from build123d import *

# Parameters (mm, degrees)
FILLET1_R     = 1
CHAMFER1_SIZE = 1


with BuildPart() as part:
    # Sketch1 → Revolve1 (revolve)
    with BuildSketch(Plane(origin=(0, 0, 0), x_dir=(0, 0, -1), z_dir=(1, 0, 0)), mode=Mode.PRIVATE) as revolve1_sk:
        with BuildLine():
            Line((-55, 0), (358, 0))
            Line((358, 0), (358, 30.75))
            ThreePointArc((358, 30.75), (357.69848481, 34.992640687), (356.8, 39.15))
            Line((356.8, 39.15), (331.5, 40.033495468))
            Line((331.5, 40.033495468), (331.5, 42.5))
            Line((331.5, 42.5), (318.5, 42.5))
            Line((318.5, 42.5), (318.5, 65))
            Line((318.5, 65), (200.002907484, 65))
            Line((200.002907484, 65), (200.002907484, 55))
            Line((200.002907484, 55), (148, 55))
            Line((148, 55), (148, 66))
            Line((148, 66), (80, 66))
            Line((80, 66), (80, 63))
            Line((80, 63), (74, 63))
            Line((74, 63), (74, 66))
            Line((74, 66), (57, 66))
            Line((57, 66), (57, 65))
            Line((57, 65), (42, 65))
            Line((42, 65), (42, 47))
            Line((42, 47), (22, 45.5))
            Line((22, 45.5), (2, 45.5))
            Line((2, 45.5), (2, 22.5))
            Line((2, 22.5), (0, 22.5))
            Line((0, 22.5), (0, 17.5))
            Line((0, 17.5), (-55, 17.5))
            Line((-55, 17.5), (-55, 0))
        make_face()
    revolve(revolve1_sk.sketch.rotate(Axis((0, 0, 61.708002771), (0, 0, -1)), 90), axis=Axis((0, 0, 61.708002771), (0, 0, -1)))

    # Fillet1
    fillet1_edges = [part.edges().sort_by_distance(p)[0] for p in [
        (-39.15, 0, -356.8),
    ]]
    fillet(fillet1_edges, radius=FILLET1_R)

    # Chamfer1
    chamfer1_edges = [part.edges().sort_by_distance(p)[0] for p in [
        (-17.5, 0, 55),
    ]]
    chamfer(chamfer1_edges, length=CHAMFER1_SIZE)


solid = part.part
Geometry check sheet. Reference: the model listing, model coordinates, mm. A direction names the side the tool comes from. Round coordinates to 2 decimals unless told otherwise and drop trailing zeros. Order: outer loops, then holes, each group sorted by start corner. A loop starts at its lowest first (then second) coordinate and runs counter-clockwise, first axis right, second up. Notation, with made-up numbers: M -10.5,13 L 48.5,13 A31 ccw 48.5,43 Z; hole C -2,19.5 d6. An arc over 180 degrees is marked long. Write each question's results on one line, items separated by ' | '. Start each with the question number.
1. Set-up check for faces 1 (the face through (29, 28, -331.5)), 2 (the face through (43, -20, -42)), 3 (the face through (-58.4, 24.1, -74)): record each of +Z, -Z, +X, -X, +Y, -Y from which the full face is reachable in a straight line by a thin tool's end or side.
2. Draft check along Z on faces 4 (the face through (58.4, 24.1, -80)), 5 (the face through (62, -19.52, -49.4)), 6 (the face through (0, 0, 55)). Enter one of: pulls with the +Z half, pulls with the -Z half, needs draft (parallel to the pull), parting line crosses it, or undercut.
3. Go/stop test with flat-tipped pins: P1, Ø4, axis at x = 28.5, z = -4, coming from the +Y side; P2, Ø3, axis at y = 31.5, z = -70, coming from the -X side; P3, Ø1.5, axis at y = -7, z = -66.5, coming from the -X side. Record where each tip stops, or that it passes through.
4. Material ranges on L1, parallel to Z at x = 52, y = -31.5; L2, parallel to Z at x = -37, y = 10.5; L3, parallel to Z at x = 20, y = 45, recorded low to high. Write a range as from..to.
5. Cross-section at A-A on z = -241. Record the boundary of the cut face in (x, y).
Resolved:
1) face 1: -Z | face 2: +Z | face 3: none
2) face 4: undercut | face 5: needs draft | face 6: pulls with the +Z half
3) P1: y = 36.99 | P2: x = -58.79 | P3: x = -65.7
4) L1: -318.5..-200, -148..-42 | L2: -356.99..-2 | L3: -318.5..-42
5) outline: C 0,0 d130
